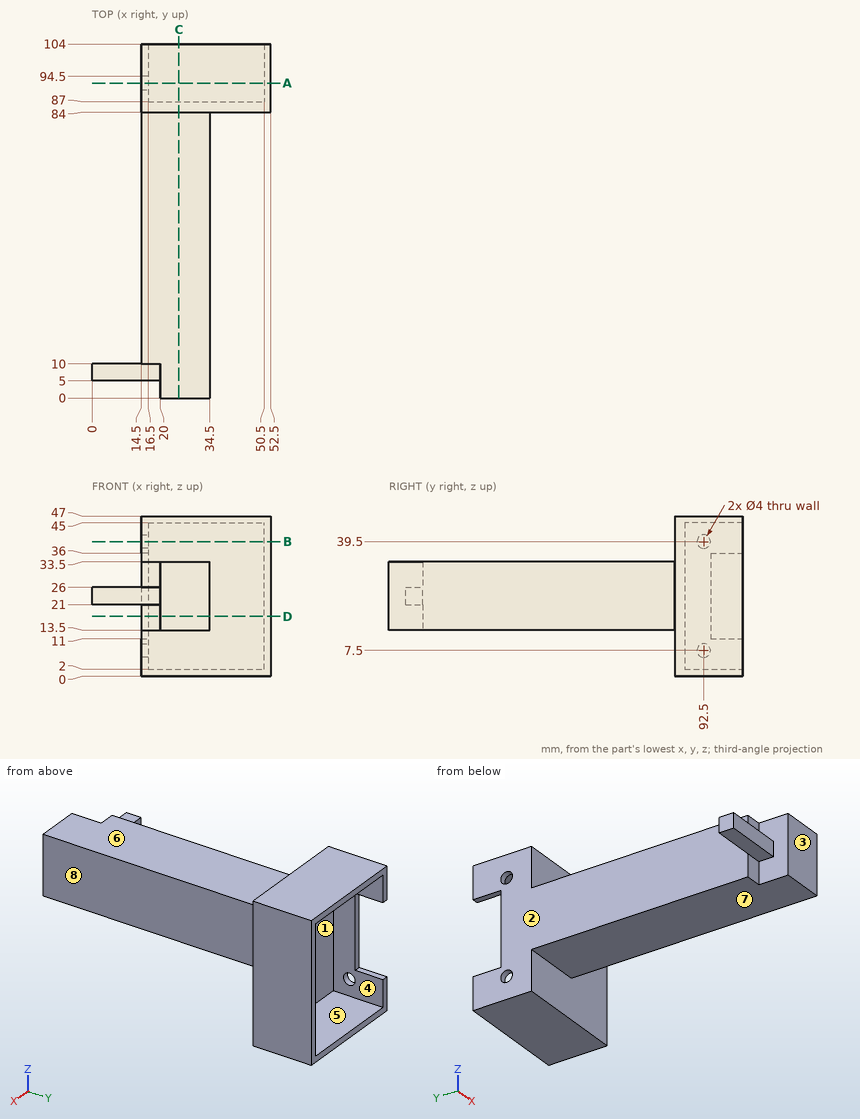
Answer from the drawing. Dimensions are ordinates in mm from the lowest x, y and z of the part. A direction names the side the tool comes from. Round coordinates to 2 decimals unless told otherwise and drop trailing zeros. Loops run counter-clockwise (first coordinate to the right, second up) from the corner with the lowest first, then second, coordinate; pieces in that order, holes last.
Q1. Section A-A on y = 92.5 is taken. Write down the section's boundary in (x, z).
Q2. Which of the six approach directions +Z, -Z, +X, -X, +Y, -Y give full straight-line access (tool end or side, diameter ignored) to the marked faces 5, 6, 7 and 8?
Q3. Section B-B on z = 39.5 is taken. Write down the section's boundary in (x, y), and give its area (3 significant figures).
Q4. Each of these flat-tipped pins is pushed along its axis until it touches: pin 1 (5 mm diameter, centred on y = 16, z = 21.5, fed in from -X); pin 2 (10 mm diameter, centred on x = 41.5, z = 29.5, fed in from +Y); pin 3 (2.5 mm diameter, centred on x = 5.5, z = 23, fed in from -Y). Where does it stop, or does it pass through?
Q5. Section C-C on x = 25.5 is taken. Write down the section's boundary in (y, z), and give its area (3 significant figures).
Q6. Determine the mould class of the marked faces 1, 2, 3 and 4 for opening direction X: released by +X, released by -X, zero draft, split by the parting line, or undercut.
Q7. Consider probe 1 along Z at (x, y) = (15, 92); probe 2 along X at (y, z) = (93, 2.5); probe 3 along Y at (x, z) = (15.7, 39.5). Determine where each line is inside the solid, lowest interval first.
Q8. Section D-D on z = 17.5 is taken. Write down the section's boundary in (x, y).
Output:
1. outline: (14.5, 0) - (52.5, 0) - (52.5, 47) - (14.5, 47) - (14.5, 41.5) - (16.5, 41.5) - (16.5, 45) - (50.5, 45) - (50.5, 2) - (16.5, 2) - (16.5, 5.5) - (14.5, 5.5) - close; (14.5, 9.5) - (16.5, 9.5) - (16.5, 37.5) - (14.5, 37.5) - close
2. face 5: +Y
2. face 6: +Z, +X, -X, -Y
2. face 7: -Z, +X, -X, -Y
2. face 8: +Z, -Z, +X, -Y
3. outline: (14.5, 84) - (52.5, 84) - (52.5, 104) - (50.5, 104) - (50.5, 87) - (16.5, 87) - (16.5, 90.5) - (14.5, 90.5) - close; (14.5, 94.5) - (16.5, 94.5) - (16.5, 104) - (14.5, 104) - close
3. area: 174 mm2
4. pin 1: stops at x = 14.5
4. pin 2: stops at y = 87
4. pin 3: stops at y = 5
5. outline: (0, 13.5) - (84, 13.5) - (84, 0) - (104, 0) - (104, 2) - (87, 2) - (87, 45) - (104, 45) - (104, 47) - (84, 47) - (84, 33.5) - (0, 33.5) - close
5. area: 1,890 mm2
6. face 1: undercut
6. face 2: released by -X
6. face 3: zero draft
6. face 4: undercut
7. probe 1: z = 0 to 5.56, 9.44 to 37.56, 41.44 to 47
7. probe 2: x = 14.5 to 16.5, 50.5 to 52.5
7. probe 3: y = 84 to 90.5, 94.5 to 104
8. outline: (14.5, 10) - (20, 10) - (20, 0) - (34.5, 0) - (34.5, 84) - (52.5, 84) - (52.5, 104) - (50.5, 104) - (50.5, 87) - (16.5, 87) - (16.5, 94.5) - (14.5, 94.5) - close
